Can you work these out from the drawing? Everything is in mm from the part's minimum corner. Round coordinates to 2 decimals unless told otherwise and drop trailing zeros. Order: outer loops, then holes, each group sorted by start corner. A loop starts at its lowest first (then second) coordinate and runs counter-clockwise, first axis right, second up. Notation, with made-up numbers: M -5.75,25.25 L 28.25,25.25 A28 cw 28.25,45.25 Z; hole C -22.75,-26 d10. An arc over 180 degrees is marked long. Write item = value, one per line. Start each with the question number.
Item 1: I want a section at C-C, the plane y = 0.7. List the corners of the cut face in (x, z) for me, plus the area to 3 significant figures.
Item 2: We'd pull the mould along Z, two halves only. Please class the marked faces 1, 2, 3 and 4: pulls with the +Z half, pulls with the -Z half, needs draft (parallel to the pull), parting line crosses it, or undercut.
Item 3: I want a section at A-A, the plane x = 5. List the corners of the cut face in (y, z) for me, plus the area to 3 significant figures.
Item 4: Please list where these lines run through material, in increasing order: L1, parallel to X at y = 1.35, z = 15; L2, parallel to Z at x = 5.75, y = 0.85; L3, parallel to X at y = 0.2, z = 15.5.
Item 5: I want a section at B-B, the plane z = 15. List the corners of the cut face in (x, y) for me, plus the area to 3 significant figures.
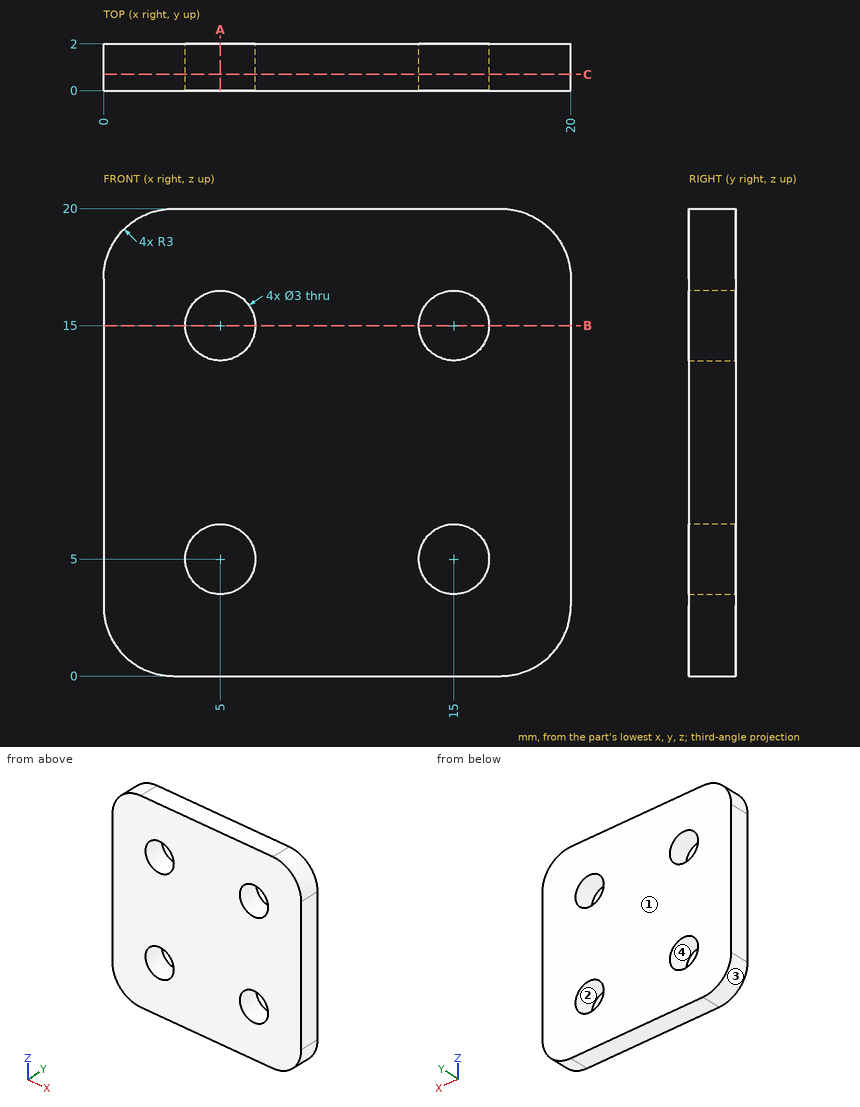
Filled in:
q1.outline = M 0,3 A3 ccw 3,0 L 17,0 A3 ccw 20,3 L 20,17 A3 ccw 17,20 L 3,20 A3 ccw 0,17 Z; hole C 5,5 d3; hole C 5,15 d3; hole C 15,5 d3; hole C 15,15 d3
q1.area = 364 mm^2
q2.face_1 = needs draft
q2.face_2 = undercut
q2.face_3 = pulls with the -Z half
q2.face_4 = undercut
q3.outline = M 0,0 L 2,0 L 2,3.5 L 0,3.5 Z; M 0,6.5 L 2,6.5 L 2,13.5 L 0,13.5 Z; M 0,16.5 L 2,16.5 L 2,20 L 0,20 Z
q3.area = 28.0 mm^2
q4.L1 = 0 to 3.5, 6.5 to 13.5, 16.5 to 20
q4.L2 = 0 to 3.7, 6.3 to 13.7, 16.3 to 20
q4.L3 = 0 to 3.59, 6.41 to 13.59, 16.41 to 20
q5.outline = M 0,0 L 3.5,0 L 3.5,2 L 0,2 Z; M 6.5,0 L 13.5,0 L 13.5,2 L 6.5,2 Z; M 16.5,0 L 20,0 L 20,2 L 16.5,2 Z
q5.area = 28.0 mm^2
